```python
from build123d import *

# Parameters (mm, degrees)
SKETCH_1_W      = 76
SKETCH_1_H      = 58
SKETCH_1_R      = 1.5
EXTRUDE_1_DEPTH = 1.8
SKETCH_2_W      = 12
SKETCH_2_H      = 8
SKETCH_2_W_2    = 8
SKETCH_2_H_2    = 12
EXTRUDE_2_DEPTH = 8
SKETCH_3_W      = 10
SKETCH_3_H      = 4
SKETCH_3_W_2    = 4
SKETCH_3_H_2    = 10
EXTRUDE_3_DEPTH = 4
SKETCH_4_R      = 7.5
EXTRUDE_4_DEPTH = 30
FILLET_1_R      = 5


with BuildPart() as part:
    # 草图1 → 凸台-拉伸1 (new body)
    with BuildSketch(Plane.XY):
        Rectangle(SKETCH_1_W, SKETCH_1_H)
        with Locations((-32.75, 24.75)):
            Circle(SKETCH_1_R, mode=Mode.SUBTRACT)
        with Locations((-32.75, -24.75)):
            Circle(SKETCH_1_R, mode=Mode.SUBTRACT)
        with Locations((32.75, -24.75)):
            Circle(SKETCH_1_R, mode=Mode.SUBTRACT)
        with Locations((32.75, 24.75)):
            Circle(SKETCH_1_R, mode=Mode.SUBTRACT)
    extrude(amount=EXTRUDE_1_DEPTH)

    # 草图2 → 凸台-拉伸2 (add)
    with BuildSketch(Plane.XY.offset(1.8)):
        with Locations((34, 18)):
            Rectangle(SKETCH_2_W, SKETCH_2_H)
        with Locations((34, 3)):
            Rectangle(SKETCH_2_W, SKETCH_2_H)
        with Locations((34, -12)):
            Rectangle(SKETCH_2_W, SKETCH_2_H)
        with Locations((-7.25, -25)):
            Rectangle(SKETCH_2_W_2, SKETCH_2_H_2)
        with Locations((20.75, -25)):
            Rectangle(SKETCH_2_W_2, SKETCH_2_H_2)
    extrude(amount=EXTRUDE_2_DEPTH)

    # 草图3 → 凸台-拉伸3 (add)
    with BuildSketch(Plane.XY.offset(1.8)):
        with Locations((-24.75, 27)):
            Rectangle(SKETCH_3_W, SKETCH_3_H)
        with Locations((-13.75, 27)):
            Rectangle(SKETCH_3_W, SKETCH_3_H)
        with Locations((-36, 7.75)):
            Rectangle(SKETCH_3_W_2, SKETCH_3_H_2)
    extrude(amount=EXTRUDE_3_DEPTH)

    # 草图4 → 凸台-拉伸4 (add)
    with BuildSketch(Plane.XY.offset(1.8)):
        with Locations(Location((4.75, -21, 0), (0, 0, 180))):
            Circle(SKETCH_4_R)
    extrude(amount=EXTRUDE_4_DEPTH)

    # 圆角1
    fillet_1_edges = [part.edges().sort_by_distance(p)[0] for p in [
        (38, -29, 0.9),
        (-38, -29, 0.9),
        (-38, 29, 0.9),
        (38, 29, 0.9),
    ]]
    fillet(fillet_1_edges, radius=FILLET_1_R)


solid = part.part
```
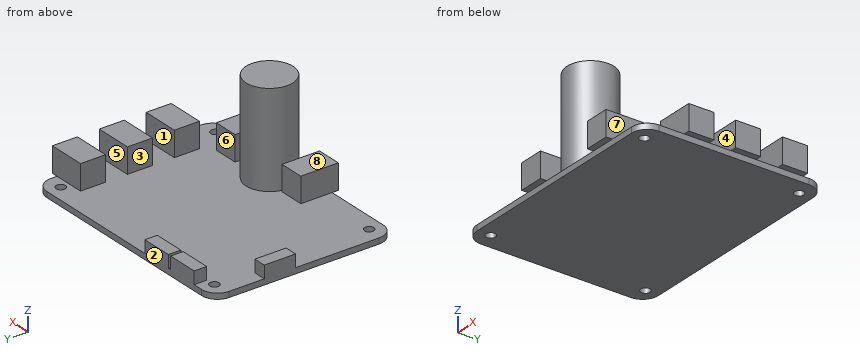
Input: part model. Units: mm. Frame: model coordinates. Face numbers are marked on the shaded views. A direction names the side the tool comes from. Coordinates: 2 decimals unless noted, no trailing zeros. Write each loop counter-clockwise with the first axis right and the second up, starting at its lowest first coordinate (ties: lowest second). Pieces come first, ordered by that corner, then holes.
1) Material intervals for line 1 along Y through (x, z) = (-32.75, 0.7); line 2 along Z through (x, y) = (-29, 8.5); line 3 along X through (y, z) = (21, 5), sorted ascending.
2) Set-up query: the marked faces 4, 5, 6, 7 and 8. Return all of +Z, -Z, +X, -X, +Y, -Y with unobstructed straight access to the full face (end or side cutting, diameter ignored); none if empty.
3) Section C-C on x = 4.75. Output: boundary loops of the cut face in (y, z), and give its area (3 significant figures).
4) Pin query (flat end, axial travel): pin 1 Ø0.6 at (x, y) = (39.5, 1.5) entering from -Z; pin 2 Ø1.2 at (y, z) = (7.5, 3.5) entering from +X; pin 3 Ø9 at (x, z) = (33, 6.5) entering from -Y; pin 4 Ø4 at (y, z) = (-23, 5) entering from +X. Return the tip coordinate at first contact, or that it passes through.
5) Section A-A on z = 7.5. Output: boundary loops of the cut face in (x, y).
6) Section D-D on z = 23.5. Output: boundary loops of the cut face in (x, y), and give its area (3 significant figures).
7) Section B-B on y = 1.5. Output: boundary loops of the cut face in (x, z), and give its area (3 significant figures).
8) Mould query, pull axis Y, two halves, no side actions, for the marked faces 1, 2 and 3. Classes: pulls with the +Y half, pulls with the -Y half, needs draft (parallel to the pull), parting line crosses it, or undercut.
Check result:
1. line 1: y = -29 to -26.25, -23.25 to 23.25, 26.25 to 29
1. line 2: z = 0 to 1.8
1. line 3: x = 28 to 40
2. face 4: +Z, +X, -X
2. face 5: +Z, +X
2. face 6: +Z, +X, +Y
2. face 7: +Z, +X, +Y, -Y
2. face 8: +Z, -X, +Y, -Y
3. outline: (-29, 0) - (29, 0) - (29, 1.8) - (-13.5, 1.8) - (-13.5, 31.8) - (-28.5, 31.8) - (-28.5, 1.8) - (-29, 1.8) - close
3. area: 554 mm2
4. pin 1: stops at z = 1.8
4. pin 2: stops at x = 40
4. pin 3: stops at y = -16
4. pin 4: stops at x = 24.75
5. outline: (-11.25, -31) - (-3.25, -31) - (-3.25, -19) - (-11.25, -19) - close; circle Ø15 at (4.75, -21); (16.75, -31) - (24.75, -31) - (24.75, -19) - (16.75, -19) - close; (28, -16) - (40, -16) - (40, -8) - (28, -8) - close; (28, -1) - (40, -1) - (40, 7) - (28, 7) - close; (28, 14) - (40, 14) - (40, 22) - (28, 22) - close
6. outline: circle Ø15 at (4.75, -21)
6. area: 177 mm2
7. outline: (-38, 0) - (38, 0) - (38, 1.8) - (40, 1.8) - (40, 9.8) - (28, 9.8) - (28, 1.8) - (-38, 1.8) - close
7. area: 233 mm2
8. face 1: undercut
8. face 2: pulls with the +Y half
8. face 3: needs draft
